Source: CAD feature listing. Evaluate the final solid. Frame: model axes, mm. A direction names the side the tool comes from. Coordinates: 2 decimals unless noted, no trailing zeros. Write each loop counter-clockwise with the first axis right and the second up, starting at its lowest first coordinate (ties: lowest second). Pieces come first, ordered by that corner, then holes. Notation, with made-up numbers: (55, 21) - (83, 21) arc R21 cw to (83, 54) - close; hole circle Ø9 at (9, 40). An arc over 180 degrees is marked (long way). One line per question, with ' | ' between items.
from build123d import *

# Parameters (mm, degrees)
SKETCH_1_W      = 60
SKETCH_1_H      = 50
SKETCH_1_R      = 1.6
EXTRUDE_1_DEPTH = 3
FILLET_1_R      = 2
FILLET_2_R      = 2


with BuildPart() as part:
    # 草图1 → 凸台-拉伸1 (new body)
    with BuildSketch(Plane(origin=(0, 0, 0), x_dir=(1, 0, 0), z_dir=(0, 1, 0))):
        Rectangle(SKETCH_1_W, SKETCH_1_H)
        with Locations((-25, 21)):
            Circle(SKETCH_1_R, mode=Mode.SUBTRACT)
        with Locations((25, 21)):
            Circle(SKETCH_1_R, mode=Mode.SUBTRACT)
        with Locations((25, -21)):
            Circle(SKETCH_1_R, mode=Mode.SUBTRACT)
        with Locations((-25, -21)):
            Circle(SKETCH_1_R, mode=Mode.SUBTRACT)
        Polygon((-25, 17.579062635), (-3.905124838, 0), (-25, -17.579062635), align=None, mode=Mode.SUBTRACT)
        Polygon((25, 17.579062635), (25, -17.579062635), (3.905124838, 0), align=None, mode=Mode.SUBTRACT)
        Polygon((-20.094875162, -20), (0, -3.254270698), (20.094875162, -20), align=None, mode=Mode.SUBTRACT)
        Polygon((20.094875162, 20), (0, 3.254270698), (-20.094875162, 20), align=None, mode=Mode.SUBTRACT)
    extrude(amount=EXTRUDE_1_DEPTH)

    # 圆角1
    fillet_1_edges = [part.edges().sort_by_distance(p)[0] for p in [
        (30, 1.5, 25),
        (-30, 1.5, 25),
        (-30, 1.5, -25),
        (30, 1.5, -25),
    ]]
    fillet(fillet_1_edges, radius=FILLET_1_R)

    # 圆角2
    fillet_2_edges = [part.edges().sort_by_distance(p)[0] for p in [
        (-25, 1.5, -17.579062635),
        (-25, 1.5, 17.579062635),
        (-3.905124838, 1.5, 0),
        (-20.094875162, 1.5, 20),
        (20.094875162, 1.5, 20),
        (0, 1.5, 3.254270698),
        (3.905124838, 1.5, 0),
        (25, 1.5, 17.579062635),
        (25, 1.5, -17.579062635),
        (20.094875162, 1.5, -20),
        (-20.094875162, 1.5, -20),
        (0, 1.5, -3.254270698),
    ]]
    fillet(fillet_2_edges, radius=FILLET_2_R)


solid = part.part
Item 1: Ray query, line 1 along X through (y, z) = (2.1, 21); line 2 along X through (y, z) = (0.7, -8.5); line 3 along Z through (x, y) = (-9, 2.5). Return the intervals inside material, ascending. Write a range as [from, to].
Check sheet entries:
line 1: [-30, -26.6], [-23.4, 23.4], [26.6, 30] | line 2: [-30, -25], [-14.11, -6.29], [6.29, 14.11], [25, 30] | line 3: [-25, -20], [-10.75, -4.25], [4.25, 10.75], [20, 25]
Item 2: Access query for faces 4 (the face through (30, 1, 0)), 5 (the face through (0.019, 1.521, 3.858)). Directions: +Z, -Z, +X, -X, +Y, -Y. A direction counts if a zero-diameter tool reaches every point of the face in a straight line with its end or side. Return the directions, or none.
Check sheet entries:
face 4: +Z, -Z, +X, +Y, -Y | face 5: +Y, -Y
Item 3: Cut plane C-C on x = -8.5. Return loops of the section in (y, z), and give its area (3 significant figures).
Check sheet entries:
outline: (0, -25) - (3, -25) - (3, -20) - (0, -20) - close; (0, -10.34) - (3, -10.34) - (3, -3.83) - (0, -3.83) - close; (0, 3.83) - (3, 3.83) - (3, 10.34) - (0, 10.34) - close; (0, 20) - (3, 20) - (3, 25) - (0, 25) - close | area: 69.1 mm²
Item 4: Mould query, pull axis Z, two halves, no side actions, for faces 1 (the face through (0, 1, 25)), 2 (the face through (-30, 1, 0)), 3 (the face through (13.622, 1.479, -8.098)). Classes: pulls with the +Z half, pulls with the -Z half, needs draft (parallel to the pull), parting line crosses it, or undercut.
Check sheet entries:
face 1: pulls with the +Z half | face 2: needs draft | face 3: undercut
Item 5: Cut plane A-A on x = 2. Return loops of the section in (y, z).
Check sheet entries:
outline: (0, -25) - (3, -25) - (3, -20) - (0, -20) - close; (0, -4.92) - (3, -4.92) - (3, 4.92) - (0, 4.92) - close; (0, 20) - (3, 20) - (3, 25) - (0, 25) - close
Item 6: Cut plane B-B on z = 21. Return loops of the section in (x, y).
Check sheet entries:
outline: (-30, 0) - (-26.6, 0) - (-26.6, 3) - (-30, 3) - close; (-23.4, 0) - (23.4, 0) - (23.4, 3) - (-23.4, 3) - close; (26.6, 0) - (30, 0) - (30, 3) - (26.6, 3) - close
Item 7: Pin query (flat end, axial travel): pin 1 Ø3.5 at (x, z) = (25, 21) entering from +Y; pin 2 Ø2.5 at (x, z) = (25, -21) entering from -Y. Return the tip coordinate at first contact, or that it passes through.
Check sheet entries:
pin 1: y = 3 | pin 2: through
Item 8: Cut plane D-D on z = 10. Return loops of the section in (x, y), and give its area (3 significant figures).
Check sheet entries:
outline: (-30, 0) - (-25, 0) - (-25, 3) - (-30, 3) - close; (-15.91, 0) - (-8.09, 0) - (-8.09, 3) - (-15.91, 3) - close; (8.09, 0) - (15.91, 0) - (15.91, 3) - (8.09, 3) - close; (25, 0) - (30, 0) - (30, 3) - (25, 3) - close | area: 76.9 mm²
